Geometry check sheet. Reference: the model listing, model coordinates, mm. Round coordinates to 2 decimals unless told otherwise and drop trailing zeros. Write each question's results on one line, items separated by ' | '.
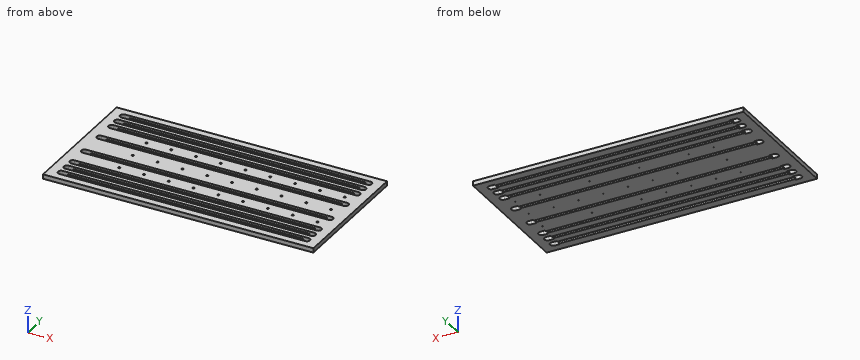
```python
from build123d import *

# Parameters (mm, degrees)
F1_W     = 1091
F1_H     = 542
F1_R     = 4
F2_DEPTH = 18
F1_R_2   = 1.5
F1_W_2   = 951
F1_H_2   = 6
F1_H_3   = 5
F3_DEPTH = 9


with BuildPart() as f2:
    # F1 (on face) → F2 (new body)
    with BuildSketch(Plane.XY):
        with Locations((545.5, 271)):
            Rectangle(F1_W, F1_H)
        with Locations((214, 171)):
            Circle(F1_R, mode=Mode.SUBTRACT)
        with Locations((314, 171)):
            Circle(F1_R, mode=Mode.SUBTRACT)
        with Locations((414, 171)):
            Circle(F1_R, mode=Mode.SUBTRACT)
        with Locations((514, 171)):
            Circle(F1_R, mode=Mode.SUBTRACT)
        with BuildLine():
            Line((70, 30.25), (50, 30.25))
            ThreePointArc((50, 30.25), (37.5, 42.75), (50, 55.25))
            Line((50, 55.25), (70, 55.25))
            Line((70, 55.25), (1021, 55.25))
            Line((1021, 55.25), (1041, 55.25))
            ThreePointArc((1041, 55.25), (1053.5, 42.75), (1041, 30.25))
            Line((1041, 30.25), (1021, 30.25))
            Line((1021, 30.25), (70, 30.25))
        make_face(mode=Mode.SUBTRACT)
        with BuildLine():
            Line((70, 73), (50, 73))
            ThreePointArc((50, 73), (37.5, 85.5), (50, 98))
            Line((50, 98), (70, 98))
            Line((70, 98), (1021, 98))
            Line((1021, 98), (1041, 98))
            ThreePointArc((1041, 98), (1053.5, 85.5), (1041, 73))
            Line((1041, 73), (1021, 73))
            Line((1021, 73), (70, 73))
        make_face(mode=Mode.SUBTRACT)
        with BuildLine():
            Line((70, 115.75), (50, 115.75))
            ThreePointArc((50, 115.75), (37.5, 128.25), (50, 140.75))
            Line((50, 140.75), (70, 140.75))
            Line((70, 140.75), (1021, 140.75))
            Line((1021, 140.75), (1041, 140.75))
            ThreePointArc((1041, 140.75), (1053.5, 128.25), (1041, 115.75))
            Line((1041, 115.75), (1021, 115.75))
            Line((1021, 115.75), (70, 115.75))
        make_face(mode=Mode.SUBTRACT)
        with Locations((614, 171)):
            Circle(F1_R, mode=Mode.SUBTRACT)
        with Locations((714, 171)):
            Circle(F1_R, mode=Mode.SUBTRACT)
        with Locations((814, 171)):
            Circle(F1_R, mode=Mode.SUBTRACT)
        with BuildLine():
            Line((70, 202.061247), (50, 202.061247))
            ThreePointArc((50, 202.061247), (37.5, 214.561247), (50, 227.061247))
            Line((50, 227.061247), (70, 227.061247))
            Line((70, 227.061247), (1021, 227.061247))
            Line((1021, 227.061247), (1041, 227.061247))
            ThreePointArc((1041, 227.061247), (1053.5, 214.561247), (1041, 202.061247))
            Line((1041, 202.061247), (1021, 202.061247))
            Line((1021, 202.061247), (70, 202.061247))
        make_face(mode=Mode.SUBTRACT)
        with Locations((914, 171)):
            Circle(F1_R, mode=Mode.SUBTRACT)
        with Locations((1014, 171)):
            Circle(F1_R, mode=Mode.SUBTRACT)
        with Locations((214, 271)):
            Circle(F1_R, mode=Mode.SUBTRACT)
        with Locations((214, 371)):
            Circle(F1_R, mode=Mode.SUBTRACT)
        with Locations((314, 271)):
            Circle(F1_R, mode=Mode.SUBTRACT)
        with Locations((414, 271)):
            Circle(F1_R, mode=Mode.SUBTRACT)
        with Locations((514, 271)):
            Circle(F1_R, mode=Mode.SUBTRACT)
        with Locations((314, 371)):
            Circle(F1_R, mode=Mode.SUBTRACT)
        with Locations((414, 371)):
            Circle(F1_R, mode=Mode.SUBTRACT)
        with Locations((514, 371)):
            Circle(F1_R, mode=Mode.SUBTRACT)
        with Locations((614, 271)):
            Circle(F1_R, mode=Mode.SUBTRACT)
        with BuildLine():
            Line((70, 314.938753), (50, 314.938753))
            ThreePointArc((50, 314.938753), (37.5, 327.438753), (50, 339.938753))
            Line((50, 339.938753), (70, 339.938753))
            Line((70, 339.938753), (1021, 339.938753))
            Line((1021, 339.938753), (1041, 339.938753))
            ThreePointArc((1041, 339.938753), (1053.5, 327.438753), (1041, 314.938753))
            Line((1041, 314.938753), (1021, 314.938753))
            Line((1021, 314.938753), (70, 314.938753))
        make_face(mode=Mode.SUBTRACT)
        with Locations((714, 271)):
            Circle(F1_R, mode=Mode.SUBTRACT)
        with Locations((814, 271)):
            Circle(F1_R, mode=Mode.SUBTRACT)
        with Locations((614, 371)):
            Circle(F1_R, mode=Mode.SUBTRACT)
        with Locations((714, 371)):
            Circle(F1_R, mode=Mode.SUBTRACT)
        with Locations((814, 371)):
            Circle(F1_R, mode=Mode.SUBTRACT)
        with Locations((914, 271)):
            Circle(F1_R, mode=Mode.SUBTRACT)
        with Locations((1014, 271)):
            Circle(F1_R, mode=Mode.SUBTRACT)
        with Locations((914, 371)):
            Circle(F1_R, mode=Mode.SUBTRACT)
        with Locations((1014, 371)):
            Circle(F1_R, mode=Mode.SUBTRACT)
        with BuildLine():
            Line((70, 401.25), (50, 401.25))
            ThreePointArc((50, 401.25), (37.5, 413.75), (50, 426.25))
            Line((50, 426.25), (70, 426.25))
            Line((70, 426.25), (1021, 426.25))
            Line((1021, 426.25), (1041, 426.25))
            ThreePointArc((1041, 426.25), (1053.5, 413.75), (1041, 401.25))
            Line((1041, 401.25), (1021, 401.25))
            Line((1021, 401.25), (70, 401.25))
        make_face(mode=Mode.SUBTRACT)
        with BuildLine():
            Line((70, 444), (50, 444))
            ThreePointArc((50, 444), (37.5, 456.5), (50, 469))
            Line((50, 469), (70, 469))
            Line((70, 469), (1021, 469))
            Line((1021, 469), (1041, 469))
            ThreePointArc((1041, 469), (1053.5, 456.5), (1041, 444))
            Line((1041, 444), (1021, 444))
            Line((1021, 444), (70, 444))
        make_face(mode=Mode.SUBTRACT)
        with BuildLine():
            Line((70, 486.75), (50, 486.75))
            ThreePointArc((50, 486.75), (37.5, 499.25), (50, 511.75))
            Line((50, 511.75), (70, 511.75))
            Line((70, 511.75), (1021, 511.75))
            Line((1021, 511.75), (1041, 511.75))
            ThreePointArc((1041, 511.75), (1053.5, 499.25), (1041, 486.75))
            Line((1041, 486.75), (1021, 486.75))
            Line((1021, 486.75), (70, 486.75))
        make_face(mode=Mode.SUBTRACT)
    extrude(amount=F2_DEPTH)

    # F1 (on face) → F3 (join)
    with BuildSketch(Plane.XY):
        with Locations((414, 371)):
            Circle(F1_R)
        with Locations((414, 371)):
            Circle(F1_R_2, mode=Mode.SUBTRACT)
        with Locations((314, 371)):
            Circle(F1_R)
        with Locations((314, 371)):
            Circle(F1_R_2, mode=Mode.SUBTRACT)
        with Locations((214, 371)):
            Circle(F1_R)
        with Locations((214, 371)):
            Circle(F1_R_2, mode=Mode.SUBTRACT)
        with Locations((214, 271)):
            Circle(F1_R)
        with Locations((214, 271)):
            Circle(F1_R_2, mode=Mode.SUBTRACT)
        with Locations((314, 271)):
            Circle(F1_R)
        with Locations((314, 271)):
            Circle(F1_R_2, mode=Mode.SUBTRACT)
        with Locations((414, 271)):
            Circle(F1_R)
        with Locations((414, 271)):
            Circle(F1_R_2, mode=Mode.SUBTRACT)
        with Locations((514, 271)):
            Circle(F1_R)
        with Locations((514, 271)):
            Circle(F1_R_2, mode=Mode.SUBTRACT)
        with Locations((614, 271)):
            Circle(F1_R)
        with Locations((614, 271)):
            Circle(F1_R_2, mode=Mode.SUBTRACT)
        with Locations((714, 271)):
            Circle(F1_R)
        with Locations((714, 271)):
            Circle(F1_R_2, mode=Mode.SUBTRACT)
        with Locations((814, 271)):
            Circle(F1_R)
        with Locations((814, 271)):
            Circle(F1_R_2, mode=Mode.SUBTRACT)
        with Locations((914, 271)):
            Circle(F1_R)
        with Locations((914, 271)):
            Circle(F1_R_2, mode=Mode.SUBTRACT)
        with Locations((1014, 271)):
            Circle(F1_R)
        with Locations((1014, 271)):
            Circle(F1_R_2, mode=Mode.SUBTRACT)
        with Locations((1014, 171)):
            Circle(F1_R)
        with Locations((1014, 171)):
            Circle(F1_R_2, mode=Mode.SUBTRACT)
        with Locations((914, 171)):
            Circle(F1_R)
        with Locations((914, 171)):
            Circle(F1_R_2, mode=Mode.SUBTRACT)
        with Locations((814, 171)):
            Circle(F1_R)
        with Locations((814, 171)):
            Circle(F1_R_2, mode=Mode.SUBTRACT)
        with Locations((714, 171)):
            Circle(F1_R)
        with Locations((714, 171)):
            Circle(F1_R_2, mode=Mode.SUBTRACT)
        with Locations((614, 171)):
            Circle(F1_R)
        with Locations((614, 171)):
            Circle(F1_R_2, mode=Mode.SUBTRACT)
        with Locations((514, 171)):
            Circle(F1_R)
        with Locations((514, 171)):
            Circle(F1_R_2, mode=Mode.SUBTRACT)
        with Locations((414, 171)):
            Circle(F1_R)
        with Locations((414, 171)):
            Circle(F1_R_2, mode=Mode.SUBTRACT)
        with Locations((314, 171)):
            Circle(F1_R)
        with Locations((314, 171)):
            Circle(F1_R_2, mode=Mode.SUBTRACT)
        with Locations((214, 171)):
            Circle(F1_R)
        with Locations((214, 171)):
            Circle(F1_R_2, mode=Mode.SUBTRACT)
        with Locations((1014, 371)):
            Circle(F1_R)
        with Locations((1014, 371)):
            Circle(F1_R_2, mode=Mode.SUBTRACT)
        with Locations((914, 371)):
            Circle(F1_R)
        with Locations((914, 371)):
            Circle(F1_R_2, mode=Mode.SUBTRACT)
        with Locations((814, 371)):
            Circle(F1_R)
        with Locations((814, 371)):
            Circle(F1_R_2, mode=Mode.SUBTRACT)
        with Locations((714, 371)):
            Circle(F1_R)
        with Locations((714, 371)):
            Circle(F1_R_2, mode=Mode.SUBTRACT)
        with Locations((614, 371)):
            Circle(F1_R)
        with Locations((614, 371)):
            Circle(F1_R_2, mode=Mode.SUBTRACT)
        with Locations((514, 371)):
            Circle(F1_R)
        with Locations((514, 371)):
            Circle(F1_R_2, mode=Mode.SUBTRACT)
        with Locations((545.5, 508.75)):
            Rectangle(F1_W_2, F1_H_2)
        with Locations((545.5, 489.75)):
            Rectangle(F1_W_2, F1_H_2)
        with Locations((545.5, 466)):
            Rectangle(F1_W_2, F1_H_2)
        with Locations((545.5, 447)):
            Rectangle(F1_W_2, F1_H_2)
        with Locations((545.5, 423.25)):
            Rectangle(F1_W_2, F1_H_2)
        with Locations((545.5, 404.25)):
            Rectangle(F1_W_2, F1_H_2)
        with Locations((545.5, 336.938753)):
            Rectangle(F1_W_2, F1_H_2)
        with Locations((545.5, 317.938753)):
            Rectangle(F1_W_2, F1_H_2)
        with Locations((545.5, 224.061247)):
            Rectangle(F1_W_2, F1_H_2)
        with Locations((545.5, 205.061247)):
            Rectangle(F1_W_2, F1_H_2)
        with Locations((545.5, 137.75)):
            Rectangle(F1_W_2, F1_H_2)
        with Locations((545.5, 118.75)):
            Rectangle(F1_W_2, F1_H_2)
        with Locations((545.5, 95)):
            Rectangle(F1_W_2, F1_H_2)
        with Locations((545.5, 76)):
            Rectangle(F1_W_2, F1_H_2)
        with Locations((545.5, 52.75)):
            Rectangle(F1_W_2, F1_H_3)
        with Locations((545.5, 32.75)):
            Rectangle(F1_W_2, F1_H_3)
    extrude(amount=F3_DEPTH)


solid = f2.part
```
(1) Section check A-A (x = 947). Give the number of separate pieces and of enclosed holes in the cut face, then the cut area to 3 significant figures.
Answers follow:
separate pieces: 9 | enclosed holes: 0 | area: 7,000 mm²
(2) Material ranges on line 1 (Z direction, x = 200.5, y = 223); line 2 (X direction, y = 77, z = 17.25); line 3 (X direction, y = 491.5, z = 15.5), recorded low to high.
Answers follow:
line 1: 0 to 9 | line 2: 0 to 40.83, 1050.17 to 1091 | line 3: 0 to 40.19, 1050.81 to 1091
(3) Depth check by flat-ended pin: pin 1 Ø5 at (x, y) = (457, 224.5) entering from +Z; pin 2 Ø2.5 at (x, y) = (814, 271) entering from -Z. Enter the tip coordinate at first touch or a pass-through.
Answers follow:
pin 1: z = 9 | pin 2: through
